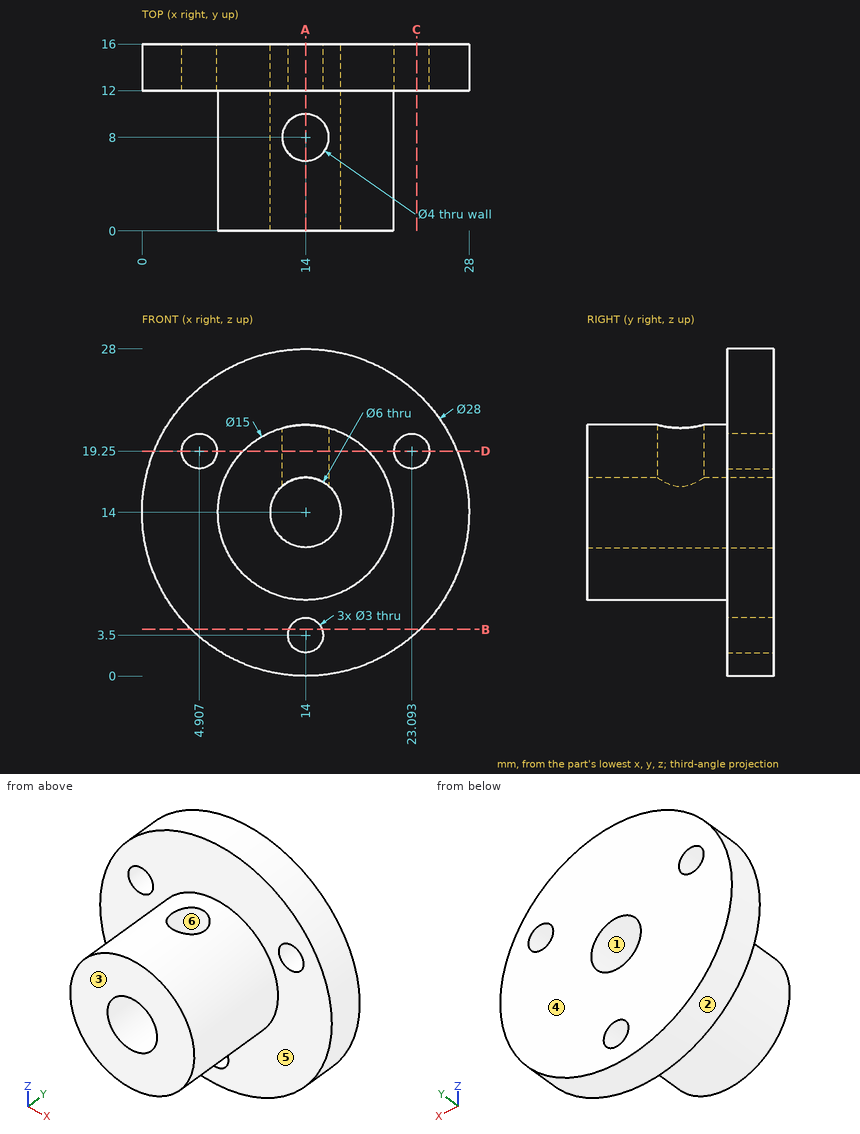
Could you check a few things on this drawing? It's one solid part, dimensions in mm from its lowest x, y, z. A direction names the side the tool comes from. Round coordinates to 2 decimals unless told otherwise and drop trailing zeros. Order: outer loops, then holes, each group sorted by start corner. A loop starts at its lowest first (then second) coordinate and runs counter-clockwise, first axis right, second up.
(1) If we mould it in two halves opening along Z, with no side actions, what happens to the marked faces 1, 2 and 3? For each: released by +Z, released by -Z, zero draft, split by the parting line, or undercut.
Response values:
face 1: undercut
face 2: split by the parting line
face 3: zero draft
(2) Imagine slicing it at C-C (x = 23.5). Write out the boundary of the cut face in (y, z), plus the area to 3 significant figures.
Response values:
outline: (12, 3.72) - (16, 3.72) - (16, 17.81) - (12, 17.81) - close; (12, 20.69) - (16, 20.69) - (16, 24.28) - (12, 24.28) - close
area: 70.7 mm2
(3) I'm going to push flat-ended pins straight in: pin 1 (1 mm diameter, centred on x = 11.5, y = 4, fed in from +Z); pin 2 (5 mm diameter, centred on x = 14, z = 14, fed in from -Y); pin 3 (1.5 mm diameter, centred on y = 8.5, z = 7, fed in from +X) (1 decimal); pin 4 (6 mm diameter, centred on y = 14.5, z = 18, fed in from -X). Where does each tip first touch, or does it pass through?
Response values:
pin 1: stops at z = 21.23
pin 2: passes through
pin 3: stops at x = 18.1
pin 4: stops at x = 0.04
(4) Imagine slicing it at A-A (x = 14). Write out the boundary of the cut face in (y, z).
Response values:
outline: (0, 6.5) - (12, 6.5) - (12, 5) - (16, 5) - (16, 11) - (0, 11) - close; (0, 17) - (6, 17) - (6, 21.5) - (0, 21.5) - close; (10, 17) - (16, 17) - (16, 28) - (12, 28) - (12, 21.5) - (10, 21.5) - close; (12, 0) - (16, 0) - (16, 2) - (12, 2) - close
(5) Which directions (+Z, -Z, +X, -X, +Y, -Y) give clear straight access to the entire face, cutting with the end or side of a thin tool? Please do the marked faces 4, 5 and 6.
Response values:
face 4: +Z, -Z, +X, -X, +Y
face 5: -Y
face 6: +Z
(6) Please list where these lines run through material, in increasing order: line 1 along X through (y, z) = (15.5, 20.5) (1 decimal); line 2 along X through (y, z) = (14.15, 19.25); line 3 along Y through (x, z) = (3.5, 17.5).
Response values:
line 1: x = 1.6 to 4.1, 5.7 to 22.3, 23.9 to 26.4
line 2: x = 1.02 to 3.41, 6.41 to 21.59, 24.59 to 26.98
line 3: y = 12 to 16
(7) Imagine slicing it at B-B (z = 4). Write out the boundary of the cut face in (x, y).
Response values:
outline: (4.2, 12) - (12.59, 12) - (12.59, 16) - (4.2, 16) - close; (15.41, 12) - (23.8, 12) - (23.8, 16) - (15.41, 16) - close
(8) Imagine slicing it at D-D (z = 19.25). Write out the boundary of the cut face in (x, y), plus the area to 3 significant figures.
Response values:
outline: (1.02, 12) - (3.41, 12) - (3.41, 16) - (1.02, 16) - close; (6.41, 12) - (8.64, 12) - (8.64, 0) - (19.36, 0) - (19.36, 12) - (21.59, 12) - (21.59, 16) - (6.41, 16) - close; (24.59, 12) - (26.98, 12) - (26.98, 16) - (24.59, 16) - close; hole circle Ø4 at (14, 8)
area: 196 mm2
